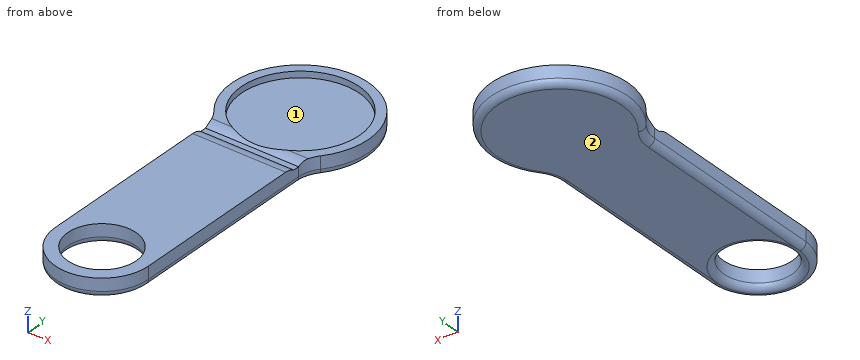
```python
from build123d import *

# Parameters (mm, degrees)
F1_DEPTH    = 3
F2_R        = 9.5
F3_DEPTH    = 1
F4_W        = 14.9929515668
F4_H        = 1
F5_DEPTH    = 0.5
F6_T1_DEPTH = 23.2845135427
F7_R        = 5.5
F8_DEPTH    = 3.0010001
F9_F1_R     = 1


# Not quite as in the source:
# - a fillet or chamfer that OpenCascade refuses, or shapes differently, is made with other operations: its cross-section is extruded or revolved along the edge and cut away or added


with BuildPart() as f1:
    # F0 (on Top) → F1 (new body)
    with BuildSketch(Plane.XY):
        with BuildLine():
            ThreePointArc((7.5, -9.9874921777), (7.781353478, -8.3338976083), (8.59375, -6.8664008722))
            ThreePointArc((8.59375, -6.8664008722), (-0.0038797807, 10.9999993158), (-8.5889042022, -6.8724613208))
            ThreePointArc((-8.5889042022, -6.8724613208), (-7.7748885732, -8.3410486079), (-7.4929515668, -9.9963073757))
            Line((-7.4929515668, -9.9963073757), (-7.4929515668, -40.6749202897))
            Line((-7.4929515668, -40.6749202897), (-7.4929515668, -41.3250797103))
            ThreePointArc((-7.4929515668, -41.3250797103), (0.162578057, -48.4982376846), (7.5, -41))
            Line((7.5, -41), (7.5, -9.9874921777))
        make_face()
    extrude(amount=F1_DEPTH)

    # F2 (on face) → F3 (cut)
    with BuildSketch(Plane.XY.offset(3)):
        Circle(F2_R)
    extrude(amount=-F3_DEPTH, mode=Mode.SUBTRACT)

    # F4 (on face) → F5 (cut)
    with BuildSketch(Plane.XY.offset(3)):
        with Locations((0.0035242166, -10.5)):
            Rectangle(F4_W, F4_H)
    extrude(amount=-F5_DEPTH, mode=Mode.SUBTRACT)

    # F6: fillet of radius 3 on 2 edges, made by hand

    # F6_s2 → F6_t1 (cut)
    with BuildSketch(Plane.YZ.offset(-11.6387325547)):
        with BuildLine():
            ThreePointArc((-12.6583123952, 3), (-11.7922869914, 2.8722813233), (-11, 2.5))
            Line((-11, 2.5), (-11, 3))
            Line((-11, 3), (-12.6583123952, 3))
        make_face()
        with BuildLine():
            ThreePointArc((-8.3416876048, 3), (-9.2077130086, 2.8722813233), (-10, 2.5))
            Line((-10, 2.5), (-10, 3))
            Line((-10, 3), (-8.3416876048, 3))
        make_face()
    extrude(amount=F6_T1_DEPTH, mode=Mode.SUBTRACT)

    # F7 (on face) → F8 (cut, through all)
    with BuildSketch(Plane.XY.offset(3)):
        with Locations((0, -41)):
            Circle(F7_R)
    extrude(amount=-F8_DEPTH, mode=Mode.SUBTRACT)

    # F9: fillet of radius 1 on 7 edges, made by hand

    # F9_f1
    f9_f1_edges = [f1.edges().sort_by_distance(p)[0] for p in [
        (-7.7748885732, -8.3410486079, 0),
        (-0.0038797807, 10.9999993158, 0),
        (-7.4929515668, -25.660693543, 0),
        (7.781353478, -8.3338976083, 0),
        (0.162578057, -48.4982376846, 0),
        (7.5, -25.4937460889, 0),
    ]]
    fillet(f9_f1_edges, radius=F9_F1_R)

    # F9_s2 → F9_t3 (revolve, cut)
    with BuildSketch(Plane.XZ.offset(41)):
        with BuildLine():
            ThreePointArc((6.5, 0), (5.7928932188, 0.2928932188), (5.5, 1))
            Line((5.5, 1), (5.48, 1))
            Line((5.48, 1), (5.48, -0.02))
            Line((5.48, -0.02), (6.5, -0.02))
            Line((6.5, -0.02), (6.5, 0))
        make_face()
    revolve(axis=Axis((0, -41, 0), (0, 0, 1)), mode=Mode.SUBTRACT)


solid = f1.part
```
Check sheet for the modelled part. Datum: model origin and axes. Units: mm. Face numbers are marked on the shaded views. Give positions to 0.01 mm unless a question says otherwise; leave off trailing zeros. Loops run counter-clockwise (first coordinate to the right, second up) from the corner with the lowest first, then second, coordinate; pieces in that order, holes last. Notation, with made-up numbers: M 32,54 L 45,54 A25 ccw 45,68 Z; hole C 9,22.5 d6. An arc over 180 degrees is marked long. Answer as CSV lines item,"result".
Item 1: Scan lines: L1, parallel to Y at x = 0, z = 2.3; L2, parallel to Y at x = 0, z = 1.6; L3, parallel to X at y = 0, z = 2.55. Record each from-to range of solid material in increasing order.
Reply:
L1,"-48.5 to -46.5, -35.5 to -9.5, 9.5 to 11"
L2,"-48.5 to -46.5, -35.5 to 11"
L3,"-11 to -9.5, 9.5 to 11"
Item 2: Sectioned sample at A-A, the plane y = -32.5. Enter the section's corners in (x, z), then the cut area to 3 significant figures.
Reply:
outline,"M -7.49,1 A1 ccw -6.49,0 L 6.5,0 A1 ccw 7.5,1 L 7.5,3 L -7.49,3 Z"
area,"44.5 mm^2"
Item 3: Draft check along Y on the marked faces 1 and 2. Enter one of: pulls with the +Y half, pulls with the -Y half, needs draft (parallel to the pull), parting line crosses it, or undercut.
Reply:
face 1,"undercut"
face 2,"needs draft"
Item 4: Depth check by flat-ended pin: pin 1 Ø1.5 at (y, z) = (-20, 1) entering from +X; pin 2 Ø5.5 at (x, y) = (-0.5, 3.5) entering from +Z; pin 3 Ø1.1 at (x, y) = (0, -10.5) entering from +Z. Enter the tip coordinate at first touch or a pass-through.
Reply:
pin 1,"x = 7.5"
pin 2,"z = 2"
pin 3,"z = 2.53"
